Print and shaded views of the part. All mm, measured from the part's lowest x, y and z. Round coordinates to 2 decimals unless told otherwise and drop trailing zeros. Loops run counter-clockwise (first coordinate to the right, second up) from the corner with the lowest first, then second, coordinate; pieces in that order, holes last. Notation, with made-up numbers: (79.25, 66) -> (128.25, 66) arc R13 ccw to (128.25, 86) -> close; hole circle Ø11 at (58.5, 24.5). An arc over 180 degrees is marked (long way). Use a Markdown table: item, result.
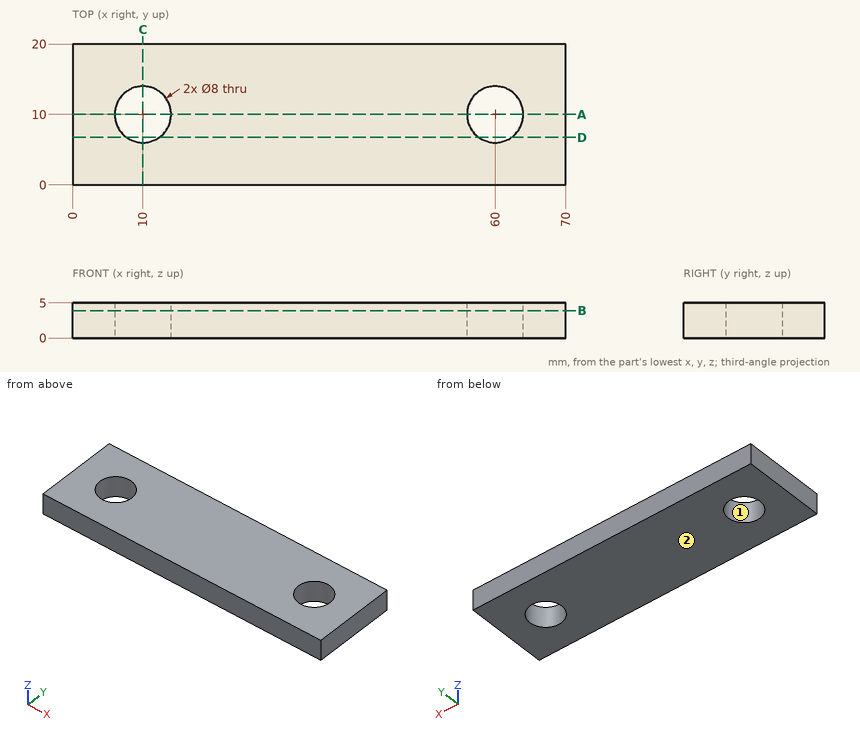
Q1. Drill centre lines: L1, parallel to X at y = 10.25, z = 4.45; L2, parallel to Y at x = 10, z = 3.2; L3, parallel to X at y = 12.25, z = 0.6. Where is each one in solid material? Low to high. Write a range as from..to.
Results list:
| item | result |
|---|---|
| L1 | x = 0..6.01, 13.99..56.01, 63.99..70 |
| L2 | y = 0..6, 14..20 |
| L3 | x = 0..6.69, 13.31..56.69, 63.31..70 |
Q2. Flat gauge pins, fed straight in: pin 1 (7 mm diameter, centred on x = 10, y = 10, fed in from +Z); pin 2 (1 mm diameter, centred on x = 39.5, z = 1.5, fed in from -Y). Where does each tip first touch, or does it go through?
Results list:
| item | result |
|---|---|
| pin 1 | passes through |
| pin 2 | stops at y = 0 |
Q3. Band-saw the part on A-A, the plane y = 10. Give the cut face in (x, z), plus the area to 3 significant figures.
Results list:
| item | result |
|---|---|
| outline | (0, 0) -> (6, 0) -> (6, 5) -> (0, 5) -> close; (14, 0) -> (56, 0) -> (56, 5) -> (14, 5) -> close; (64, 0) -> (70, 0) -> (70, 5) -> (64, 5) -> close |
| area | 270 mm² |
Q4. Band-saw the part on B-B, the plane z = 3.9. Give the cut face in (x, y).
Results list:
| item | result |
|---|---|
| outline | (0, 0) -> (70, 0) -> (70, 20) -> (0, 20) -> close; hole circle Ø8 at (10, 10); hole circle Ø8 at (60, 10) |
Q5. Pull direction X, two halves, no side cores. Call the marked faces 1 and 2: released by +X, released by -X, zero draft, split by the parting line, or undercut.
Results list:
| item | result |
|---|---|
| face 1 | undercut |
| face 2 | zero draft |
Q6. Band-saw the part on C-C, the plane x = 10. Give the cut face in (y, z), plus the area to 3 significant figures.
Results list:
| item | result |
|---|---|
| outline | (0, 0) -> (6, 0) -> (6, 5) -> (0, 5) -> close; (14, 0) -> (20, 0) -> (20, 5) -> (14, 5) -> close |
| area | 60.0 mm² |
Q7. Band-saw the part on D-D, the plane y = 6.75. Give the cut face in (x, z).
Results list:
| item | result |
|---|---|
| outline | (0, 0) -> (7.67, 0) -> (7.67, 5) -> (0, 5) -> close; (12.33, 0) -> (57.67, 0) -> (57.67, 5) -> (12.33, 5) -> close; (62.33, 0) -> (70, 0) -> (70, 5) -> (62.33, 5) -> close |
